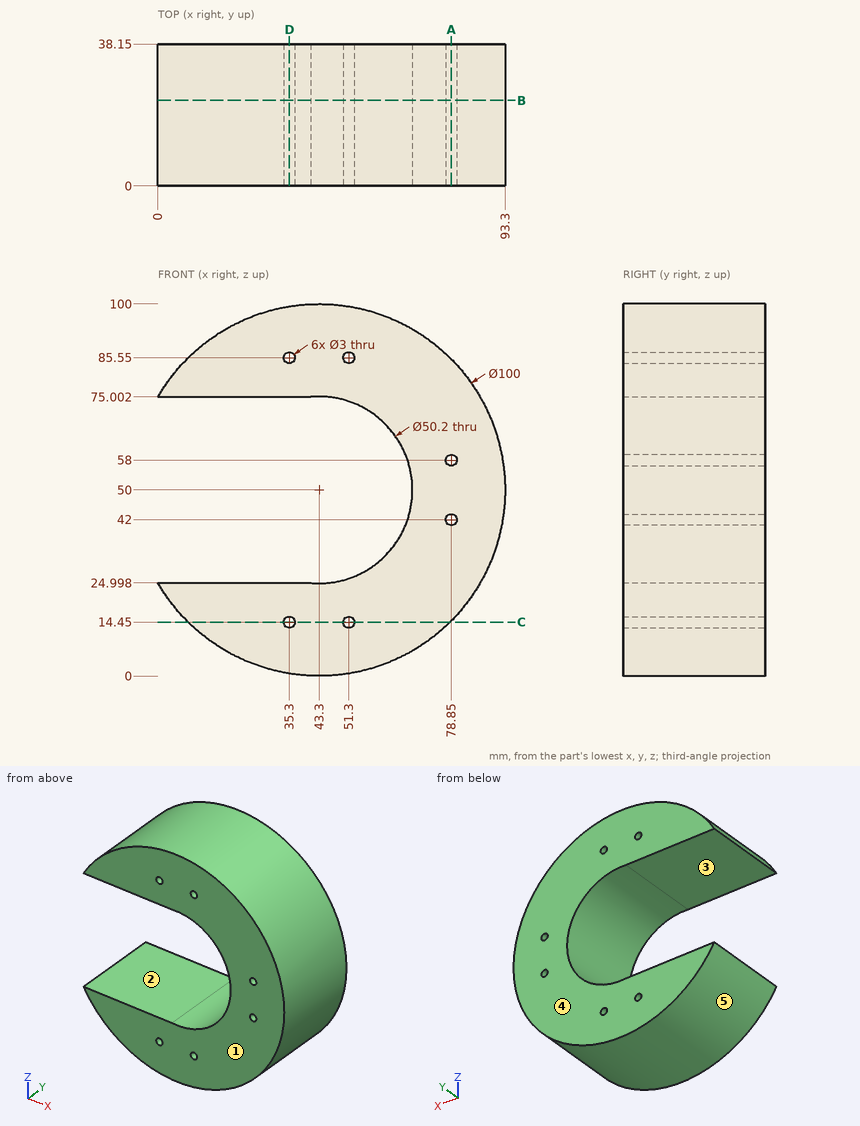
Geometry check sheet. Reference: drawing and pictorial views, mm from the part's lowest x, y, z. A direction names the side the tool comes from. Coordinates: 2 decimals unless noted, no trailing zeros. Write each loop counter-clockwise with the first axis right and the second up, starting at its lowest first coordinate (ties: lowest second). Pieces come first, ordered by that corner, then holes. Notation, with made-up numbers: (-20, -33.75) - (37, -33.75) arc R22 ccw to (37, -8.75) - close; hole circle Ø1 at (-9, 53.5). An arc over 180 degrees is marked (long way). One line per question, with ' | ' between items. Start each with the question number.
1. Material ranges on line 1 along Z through (x, y) = (51, 10); line 2 along Z through (x, y) = (77.5, 18) (1 decimal); line 3 along Z through (x, y) = (78.85, 22), recorded low to high.
2. Gauge pin test, flat ends, axial feed: P1, Ø1, axis at x = 28, y = 10.5, coming from the -Z side; P2, Ø8, axis at y = 17.5, z = 56, coming from the +X side; P3, Ø4, axis at y = 31, z = 66, coming from the +X side; P4, Ø2.5, axis at x = 35.3, z = 85.55, coming from the +Y side. Record the tip position at first contact, or that the pin passes through.
3. Section check A-A (x = 78.85). Enter the section's corners in (y, z), plus the area to 3 significant figures.
4. Section check B-B (y = 23). Enter the section's corners in (x, z).
5. Draft check along Z on the marked faces 3, 4 and 5. Enter one of: released by +Z, released by -Z, zero draft, split by the parting line, or undercut.
6. Section check D-D (x = 35.3). Enter the section's corners in (y, z).
7. Section check C-C (z = 14.45). Enter the section's corners in (x, y), plus the area to 3 significant figures.
8. Access from +Z, -Z, +X, -X, +Y, -Y to the whole of each face (thin tool, end or side, straight path). Record for the marked faces 1 and 2.
Computed values:
1) line 1: 0.6 to 12.98, 15.92 to 26.11, 73.89 to 84.08, 87.02 to 99.4 | line 2: 13.5 to 41.3, 42.7 to 57.3, 58.7 to 86.5 | line 3: 14.84 to 40.5, 43.5 to 56.5, 59.5 to 85.16
2) P1: z = 2.24 | P2: x = 93.26 | P3: x = 91.3 | P4: through
3) outline: (0, 14.84) - (38.15, 14.84) - (38.15, 40.5) - (0, 40.5) - close; (0, 43.5) - (38.15, 43.5) - (38.15, 56.5) - (0, 56.5) - close; (0, 59.5) - (38.15, 59.5) - (38.15, 85.16) - (0, 85.16) - close | area: 2,450 mm²
4) outline: (0, 25) arc R50 ccw (long way) to (0, 75) - (41.09, 75) arc R25.1 cw (long way) to (41.09, 25) - close; hole circle Ø3 at (35.3, 14.45); hole circle Ø3 at (35.3, 85.55); hole circle Ø3 at (51.3, 14.45); hole circle Ø3 at (51.3, 85.55); hole circle Ø3 at (78.85, 42); hole circle Ø3 at (78.85, 58)
5) face 3: undercut | face 4: zero draft | face 5: split by the parting line
6) outline: (0, 0.64) - (38.15, 0.64) - (38.15, 12.95) - (0, 12.95) - close; (0, 15.95) - (38.15, 15.95) - (38.15, 25) - (0, 25) - close; (0, 75) - (38.15, 75) - (38.15, 84.05) - (0, 84.05) - close; (0, 87.05) - (38.15, 87.05) - (38.15, 99.36) - (0, 99.36) - close
7) outline: (8.14, 0) - (33.8, 0) - (33.8, 38.15) - (8.14, 38.15) - close; (36.8, 0) - (49.8, 0) - (49.8, 38.15) - (36.8, 38.15) - close; (52.8, 0) - (78.46, 0) - (78.46, 38.15) - (52.8, 38.15) - close | area: 2,450 mm²
8) face 1: +Z, -Z, +X, -X, -Y | face 2: -X, +Y, -Y
